from build123d import *

# Parameters (mm, degrees)
SKETCH1_W           = 113
SKETCH1_H           = 55
BOSS_EXTRUDE2_DEPTH = 35
SKETCH3_W           = 11.6
SKETCH3_H           = 11.8
BOSS_EXTRUDE3_DEPTH = 20
SKETCH4_R           = 1.75
BOSS_EXTRUDE4_DEPTH = 15
SKETCH5_W           = 17
SKETCH5_H           = 25.5
BOSS_EXTRUDE5_DEPTH = 23
SKETCH6_R           = 3.25
BOSS_EXTRUDE6_DEPTH = 23


with BuildPart() as part:
    # Sketch1 → Boss-Extrude2 (new body)
    with BuildSketch(Plane.XY):
        with Locations((56.5, 27.5)):
            Rectangle(SKETCH1_W, SKETCH1_H)
    extrude(amount=BOSS_EXTRUDE2_DEPTH)

    # Sketch3 → Boss-Extrude3 (add)
    with BuildSketch(Plane(origin=(113, 0, 0), x_dir=(0, 0, -1), z_dir=(1, 0, 0))):
        with Locations((-17.5, 27.5)):
            Rectangle(SKETCH3_W, SKETCH3_H)
    extrude(amount=BOSS_EXTRUDE3_DEPTH)

    # Sketch4 → Boss-Extrude4 (add)
    with BuildSketch(Plane(origin=(133, 0, 0), x_dir=(0, 0, -1), z_dir=(1, 0, 0))):
        with Locations((-17.5, 27.5)):
            Circle(SKETCH4_R)
    extrude(amount=BOSS_EXTRUDE4_DEPTH)

    # Sketch5 → Boss-Extrude5 (add)
    with BuildSketch(Plane.ZY):
        with Locations((17.5, 27.5)):
            Rectangle(SKETCH5_W, SKETCH5_H)
    extrude(amount=BOSS_EXTRUDE5_DEPTH)

    # Sketch6 → Boss-Extrude6 (add)
    with BuildSketch(Plane.ZY.offset(23)):
        with Locations((17.5, 27.5)):
            Circle(SKETCH6_R)
    extrude(amount=BOSS_EXTRUDE6_DEPTH)


solid = part.part
Check sheet for the modelled part. Datum: model origin and axes. Units: mm. A direction names the side the tool comes from. Round coordinates to 2 decimals unless told otherwise and drop trailing zeros. Loops run counter-clockwise (first coordinate to the right, second up) from the corner with the lowest first, then second, coordinate; pieces in that order, holes last. Notation, with made-up numbers: (-0.5, 80.25) - (52.5, 80.25) arc R25 cw to (52.5, 116.25) - close; hole circle Ø1 at (7, 70). An arc over 180 degrees is marked (long way). Answer as CSV lines item,"result". Start each with the question number.
Item 1: Section check A-A (y = 27.5). Record the boundary of the cut face in (x, z), and give its area (3 significant figures).
Item 2: Section check B-B (z = 17.5). Record the boundary of the cut face in (x, y).
Item 3: Scan lines: line 1 (X direction, y = 45, z = 5); line 2 (Z direction, x = 115.5, y = 28.5); line 3 (Y direction, x = -12, z = 14.5). Record each from-to range of solid material in increasing order. Write a range as [from, to].
Item 4: Depth check by flat-ended pin: P1, Ø13.5, axis at x = -11, z = 20.5, coming from the +Y side; P2, Ø2, axis at y = 12.5, z = 8.5, coming from the +X side; P3, Ø3.5, axis at x = 127.5, z = 17, coming from the -Y side. Enter the tip coordinate at first touch or a pass-through.
Item 5: Section check D-D (y = 50.5). Record the boundary of the cut face in (x, z), and give its area (4 significant figures).
Item 6: Section check C-C (z = 32.5). Record the boundary of the cut face in (x, y).
Item 7: Set-up check for faces 1 (the flat face through (-11, 14.75, 17)), 2 (the flat face through (-11, 27, 26)), 3 (the flat face through (-23, 31, 15)), 4 (the flat face through (133, 29, 19)): record each of +Z, -Z, +X, -X, +Y, -Y from which the full face is reachable in a straight line by a thin tool's end or side.
Report:
1,outline,"(-46, 14.25) - (-23, 14.25) - (-23, 9) - (0, 9) - (0, 0) - (113, 0) - (113, 11.7) - (133, 11.7) - (133, 15.75) - (148, 15.75) - (148, 19.25) - (133, 19.25) - (133, 23.3) - (113, 23.3) - (113, 35) - (0, 35) - (0, 26) - (-23, 26) - (-23, 20.75) - (-46, 20.75) - close"
1,area,"4,780 mm2"
2,outline,"(-46, 24.25) - (-23, 24.25) - (-23, 14.75) - (0, 14.75) - (0, 0) - (113, 0) - (113, 21.6) - (133, 21.6) - (133, 25.75) - (148, 25.75) - (148, 29.25) - (133, 29.25) - (133, 33.4) - (113, 33.4) - (113, 55) - (0, 55) - (0, 40.25) - (-23, 40.25) - (-23, 30.75) - (-46, 30.75) - close"
3,line 1,"x = [0, 113]"
3,line 2,"z = [11.7, 23.3]"
3,line 3,"y = [14.75, 40.25]"
4,P1,"stops at y = 40.25"
4,P2,"stops at x = 113"
4,P3,"stops at y = 21.6"
5,outline,"(0, 0) - (113, 0) - (113, 35) - (0, 35) - close"
5,area,"3,955 mm2"
6,outline,"(0, 0) - (113, 0) - (113, 55) - (0, 55) - close"
7,face 1,"+Z, -Z, -X, -Y"
7,face 2,"+Z, -X, +Y, -Y"
7,face 3,"-X"
7,face 4,"+X"
